The model under review builds one solid part; all positions refer to its coordinate system, in mm. A direction names the side the tool comes from. Round coordinates to 2 decimals unless told otherwise and drop trailing zeros. Loops run counter-clockwise (first coordinate to the right, second up) from the corner with the lowest first, then second, coordinate; pieces in that order, holes last. Notation, with made-up numbers: (33.5, -26.75) -> (45.5, -26.75) arc R18 cw to (45.5, -4.75) -> close; hole circle Ø6 at (-3.75, -8.75). An arc over 180 degrees is marked (long way). Write each question's results on one line, items separated by ' | '. Start each with the question number.
Item 1: We need section D-D (y = -140.5). Give the boundary of the cut face in (x, z), and give its area (3 significant figures).
Item 2: We need section A-A (y = -62.5). Give the boundary of the cut face in (x, z), and give its area (3 significant figures).
Item 3: Mouldability with a two-part tool opening along Y and no side actions: class faces 1 (the cylindrical face through (29.3, -122.22, 43.594)), 2 (the flat face through (29, -112, 64)), 3 (the flat face through (64.4, -138, 81)) as pulls with the +Y half, pulls with the -Y half, needs draft (parallel to the pull), parting line crosses it, or undercut.
Item 4: We need section B-B (z = 127.5). Give the boundary of the cut face in (x, y).
Item 5: For L1, parallel to Y at x = 45, z = 75; L2, parallel to Y at x = 53.5, z = 123; L3, parallel to Y at x = 54.5, z = 15, list the stretches that pass through material, from the lowest coordinate up. Write a range as from..to.
Item 6: Clearance check with flat-ended pins moving along their axes: pin 1 Ø4 at (x, z) = (27.5, 40.5) entering from -Y; pin 2 Ø8 at (x, z) = (26, 119.5) entering from +Y; pin 3 Ø6 at (x, y) = (51.5, -62.5) entering from +Z; pin 4 Ø4 at (y, z) = (-113, 29) entering from -X. State where each tip first meets the part, or that it passes through.
Item 7: Tool access review of faces 4 (the flat face through (57.9, -96, 48)), 5 (the flat face through (56.7, -87, 62)), 6 (the flat face through (53.95, -130, 30)), 7 (the flat face through (56.7, -61, 20)), 8 (the flat face through (20, -99, 80)): name each direction out of +Z, -Z, +X, -X, +Y, -Y from which nothing blocks a thin tool from reaching the whole face with its end or side.
from build123d import *

# Parameters (mm, degrees)
F1_DEPTH      = 57.9
F2_DEPTH      = 64.4
F2_DEPTH_BACK = 6.5
F3_W          = 55.5
F3_H          = 23
F4_DEPTH      = 207
F5_DEPTH      = 116
F6_DEPTH      = 96
F3_W_2        = 68.5
F7_DEPTH      = 39
F8_W          = 50
F8_H          = 50
F9_DEPTH      = 40
F10_R         = 39.99999


# Not quite as in the source:
# - a fillet or chamfer is up to 0.001 mm smaller than in the source, because OpenCascade refuses the exact size


with BuildPart() as f1:
    # F0 (on Right) → F1 (new body)
    with BuildSketch(Plane.YZ):
        Polygon((-124.7912996866, 120), (-124.7912996866, 0), (-48.5912996866, 0), (-48.5912996866, 40), (-73.9912996866, 40), (-73.9912996866, 80), (-99.3912996866, 80), (-99.3912996866, 120), align=None)
    extrude(amount=F1_DEPTH)

    # F0 (on Right) → F2 (join, two sides)
    with BuildSketch(Plane.YZ) as f2_sk:
        Polygon((-150.1912996866, 160), (-150.1912996866, 0), (-124.7912996866, 0), (-124.7912996866, 120), (-124.7912996866, 160), align=None)
    extrude(amount=F2_DEPTH)
    extrude(f2_sk.sketch, amount=-F2_DEPTH_BACK)

    # F3 (on face) → F4 (cut)
    with BuildSketch(Plane.XY.offset(160)):
        with Locations((28.95, -61.2912996866)):
            Rectangle(F3_W, F3_H)
    extrude(amount=-F4_DEPTH, mode=Mode.SUBTRACT)

    # F3 (on face) → F5 (cut, through all)
    with BuildSketch(Plane.XY.offset(160)):
        with Locations((28.95, -86.6912996866)):
            Rectangle(F3_W, F3_H)
    extrude(amount=-F5_DEPTH, mode=Mode.SUBTRACT)

    # F3 (on face) → F6 (cut, through all)
    with BuildSketch(Plane.XY.offset(160)):
        with Locations((28.95, -112.0912996866)):
            Rectangle(F3_W, F3_H)
    extrude(amount=-F6_DEPTH, mode=Mode.SUBTRACT)

    # F3 (on face) → F7 (cut)
    with BuildSketch(Plane.XY.offset(160)):
        with Locations((28.95, -137.4912996866)):
            Rectangle(F3_W_2, F3_H)
    extrude(amount=-F7_DEPTH, mode=Mode.SUBTRACT)

    # F8 (on face) → F9 (cut)
    with BuildSketch(Plane.XZ.offset(150.1912996866)):
        with Locations((28.95, 30)):
            Rectangle(F8_W, F8_H)
    extrude(amount=-F9_DEPTH, mode=Mode.SUBTRACT)

    # F10 (radius 40 in the source; OpenCascade refuses exactly that, so slightly less here)
    f10_edges = [f1.edges().sort_by_distance(p)[0] for p in [
        (28.95, -110.1913, 55),
    ]]
    fillet(f10_edges, radius=F10_R)


solid = f1.part
Here are the results:
1) outline: (-6.5, 0) -> (64.4, 0) -> (64.4, 160) -> (63.2, 160) -> (63.2, 121) -> (-5.3, 121) -> (-5.3, 160) -> (-6.5, 160) -> close; hole (3.95, 5) -> (53.95, 5) -> (53.95, 53.81) -> (3.95, 53.81) -> close | area: 6,230 mm2
2) outline: (0, 0) -> (1.2, 0) -> (1.2, 40) -> (0, 40) -> close; (56.7, 0) -> (57.9, 0) -> (57.9, 40) -> (56.7, 40) -> close | area: 96.0 mm2
3) face 1: pulls with the -Y half | face 2: undercut | face 3: needs draft
4) outline: (-6.5, -150.19) -> (64.4, -150.19) -> (64.4, -124.79) -> (-6.5, -124.79) -> close; hole (-5.3, -148.99) -> (63.2, -148.99) -> (63.2, -125.99) -> (-5.3, -125.99) -> close
5) L1: y = -150.19..-123.59, -100.59..-98.19, -75.19..-73.99 | L2: y = -150.19..-148.99, -125.99..-124.79 | L3: y = -150.19..-72.79, -49.79..-48.59
6) pin 1: stops at y = -121.14 | pin 2: stops at y = -99.39 | pin 3: passes through | pin 4: stops at x = 0
7) face 4: +Z, -Z, +X, +Y | face 5: +Z | face 6: -Y | face 7: +Z, -Z | face 8: +Z, +X, -X, +Y
